Input: part model. Units: mm. Frame: model coordinates. Face numbers are marked on the shaded views. A direction names the side the tool comes from. Give positions to 0.01 mm unless a question says otherwise; leave off trailing zeros. Order: outer loops, then holes, each group sorted by start corner. A loop starts at its lowest first (then second) coordinate and runs counter-clockwise, first axis right, second up. Notation, with made-up numbers: M 75,82 L 122,82 A29 cw 122,108 Z; hole C -26.75,75.5 d6. An arc over 180 degrees is marked long. Use a Markdown table: item, result.
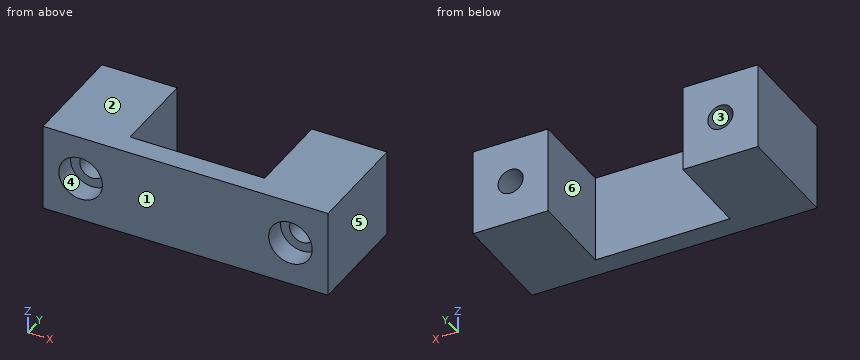
from build123d import *

# Parameters (mm, degrees)
SKETCH1_W           = 72
SKETCH1_H           = 22
BOSS_EXTRUDE1_DEPTH = 27.5
SKETCH2_W           = 34
SKETCH2_H           = 22
CUT_EXTRUDE1_DEPTH  = 22
SKETCH3_R           = 3.175
CUT_EXTRUDE2_DEPTH  = 69
SKETCH5_R           = 5.5
CUT_EXTRUDE3_DEPTH  = 5.5


with BuildPart() as part:
    # Sketch1 → Boss-Extrude1 (new body)
    with BuildSketch(Plane(origin=(0, 0, 0), x_dir=(1, 0, 0), z_dir=(0, 1, 0))):
        with Locations((36, 11)):
            Rectangle(SKETCH1_W, SKETCH1_H)
    extrude(amount=BOSS_EXTRUDE1_DEPTH)

    # Sketch2 → Cut-Extrude1 (cut)
    with BuildSketch(Plane(origin=(0, 27.5, 0), x_dir=(1, 0, 0), z_dir=(0, 1, 0))):
        with Locations((36, 11)):
            Rectangle(SKETCH2_W, SKETCH2_H)
    extrude(amount=-CUT_EXTRUDE1_DEPTH, mode=Mode.SUBTRACT)

    # Sketch3 → Cut-Extrude2 (cut)
    with BuildSketch(Plane(origin=(0, 27.5, 0), x_dir=(1, 0, 0), z_dir=(0, 1, 0))):
        with Locations(Location((9.5, 11, 0), (0, 0, 270))):
            Circle(SKETCH3_R)
        with Locations(Location((62.5, 11, 0), (0, 0, 270))):
            Circle(SKETCH3_R)
    extrude(amount=-CUT_EXTRUDE2_DEPTH, mode=Mode.SUBTRACT)

    # Sketch5 → Cut-Extrude3 (cut)
    with BuildSketch(Plane.XZ):
        with Locations(Location((9.5, -11, 0), (0, 0, 270))):
            Circle(SKETCH5_R)
        with Locations(Location((62.5, -11, 0), (0, 0, 90))):
            Circle(SKETCH5_R)
    extrude(amount=-CUT_EXTRUDE3_DEPTH, mode=Mode.SUBTRACT)


solid = part.part
1) Cut plane B-B on y = 20.75. Return loops of the section in (x, z) (3 decimals).
Response values:
| item | result |
|---|---|
| outline | M 0,-22 L 19,-22 L 19,0 L 0,0 Z; M 53,-22 L 72,-22 L 72,0 L 53,0 Z; hole C 9.5,-11 d6.35; hole C 62.5,-11 d6.35 |
2) First-contact query: pin 1 Ø7.5 at (x, z) = (62.5, -11) entering from -Y; pin 2 Ø1 at (x, z) = (43.5, -7.5) entering from +Y; pin 3 Ø3 at (x, y) = (21, 17) entering from +Z. Flat tips, straight axial feed; report the tip coordinate or a pass-through.
Response values:
| item | result |
|---|---|
| pin 1 | stops at y = 5.5 |
| pin 2 | stops at y = 5.5 |
| pin 3 | passes through |
3) Cut plane C-C on z = -11. Return loops of the section in (x, y) (3 decimals), and give its area (3 significant figures).
Response values:
| item | result |
|---|---|
| outline | M 0,0 L 4,0 L 4,5.5 L 6.325,5.5 L 6.325,27.5 L 0,27.5 Z; M 12.675,5.5 L 15,5.5 L 15,0 L 57,0 L 57,5.5 L 59.325,5.5 L 59.325,27.5 L 53,27.5 L 53,5.5 L 19,5.5 L 19,27.5 L 12.675,27.5 Z; M 65.675,5.5 L 68,5.5 L 68,0 L 72,0 L 72,27.5 L 65.675,27.5 Z |
| area | 832 mm² |
4) Cut plane A-A on x = 9.5. Return loops of the section in (y, z) (3 decimals).
Response values:
| item | result |
|---|---|
| outline | M 0,-22 L 27.5,-22 L 27.5,-14.175 L 5.5,-14.175 L 5.5,-16.5 L 0,-16.5 Z; M 0,-5.5 L 5.5,-5.5 L 5.5,-7.825 L 27.5,-7.825 L 27.5,0 L 0,0 Z |
5) Material intervals for line 1 (X direction, y = 1.55, z = -11); line 2 (X direction, y = 17, z = -11) (3 decimals); line 3 (X direction, y = 15, z = -19.5), sorted ascending. Write a range as from..to.
Response values:
| item | result |
|---|---|
| line 1 | x = 0..4, 15..57, 68..72 |
| line 2 | x = 0..6.325, 12.675..19, 53..59.325, 65.675..72 |
| line 3 | x = 0..19, 53..72 |
6) Reachability of the marked faces 4, 5 and 6 from +Z, -Z, +X, -X, +Y, -Y: full face, straight path, thin tool, end or side. Return the list, or none.
Response values:
| item | result |
|---|---|
| face 4 | -Y |
| face 5 | +Z, -Z, +X, +Y, -Y |
| face 6 | +Z, -Z, +Y |
7) Mould query, pull axis Z, two halves, no side actions, for the marked faces 1, 2 and 3. Classes: released by +Z, released by -Z, zero draft, split by the parting line, or undercut.
Response values:
| item | result |
|---|---|
| face 1 | zero draft |
| face 2 | released by +Z |
| face 3 | undercut |
8) Cut plane D-D on z = -1.75. Return loops of the section in (x, y), and give its area (3 significant figures).
Response values:
| item | result |
|---|---|
| outline | M 0,0 L 72,0 L 72,27.5 L 53,27.5 L 53,5.5 L 19,5.5 L 19,27.5 L 0,27.5 Z |
| area | 1,230 mm² |
